Work out the finished part from the listing and answer in its coordinate system (mm). A direction names the side the tool comes from. Coordinates: 2 decimals unless noted, no trailing zeros. Write each loop counter-clockwise with the first axis right and the second up, starting at its lowest first coordinate (ties: lowest second). Pieces come first, ordered by that corner, then holes. Notation, with made-up numbers: (63, 78.25) - (79, 78.25) arc R11 cw to (79, 99.25) - close; hole circle Ø6 at (59.25, 89). An arc over 180 degrees is marked (long way). One line per item, written item: value.
Autodesk Inventor part; units mm, degrees
ref_plane "YZ Plane" through (0, 0, 0) normal (1, 0, 0) x (0, 1, 0)
ref_plane "XZ Plane" through (0, 0, 0) normal (0, 1, 0) x (-1, 0, 0)
ref_plane "XY Plane" through (0, 0, 0) normal (0, 0, 1) x (1, 0, 0)
sketch "Boceto1" plane through (0, 0, 0) normal (0, 0, 1) x (1, 0, 0)
  line L0 (0, 0) -> (0, 19.566)
  line L1 (2, 65) -> (2, 21)
  line L2 (2, 21) -> (0, 19.566)
  line L3 (2, 65) -> (14.5, 65)
  line L4 (29, 0) -> (29, 19.566)
  line L5 (27, 65) -> (27, 21)
  line L6 (27, 21) -> (29, 19.566)
  line L7 (27, 65) -> (14.5, 65)
  line L8 (0, 0) -> (29, 0)
extrude "Extrusión1" add sketch "Boceto1" along normal blind 7
sketch "Boceto2" plane through (0, 0, 7) normal (0, 0, 1) x (1, 0, 0)
  line L0 (27, 65) -> (27, 21)
  line L1 (2, 65) -> (27, 65)
  line L2 (2, 21) -> (2, 65)
  line L3 (2, 65) -> (5, 65)
  line L4 (2, 65) -> (2, 26)
  line L5 (5, 26) -> (5, 65)
  line L6 (27, 65) -> (24, 65)
  line L7 (24, 65) -> (24, 44)
  line L8 (27, 65) -> (27, 26)
  line L9 (5, 26) -> (2, 26)
  line L10 (24, 26) -> (27, 26)
  line L11 (24.1227, 26) -> (22, 26)
  line L12 (22, 26) -> (22, 44)
  line L13 (22, 44) -> (24, 44)
  dimension "d7" = 18
extrude "Extrusión2" add sketch "Boceto2" along normal blind 9
sketch "Boceto3" plane through (0, 0, 7) normal (0, 0, 1) x (1, 0, 0)
  line L0 (5, 65) -> (24, 65)
  line L1 (29, 0) -> (0, 0)
  line L2 (22, 44) -> (24, 44)
  line L3 (2, 0) -> (2, 21)
  line L4 (2, 21) -> (5, 21)
  line L5 (5, 21) -> (5, 0)
  line L6 (5, 0) -> (2, 0)
  line L7 (27, 0) -> (27, 21)
  line L8 (27, 21) -> (24, 21)
  line L9 (24, 21) -> (24, 0)
  line L10 (24, 0) -> (27, 0)
  dimension "d9" = 21
extrude "Extrusión3" add sketch "Boceto3" along normal blind 5
sketch "Boceto4" plane through (0, 0, 7) normal (0, 0, 1) x (1, 0, 0)
  line L0 (29, 0) -> (0, 0)
  line L1 (7, 10) -> (15, 10)
  line L2 (15, 10) -> (15, 27)
  line L3 (15, 27) -> (7, 27)
  line L4 (7, 27) -> (7, 10)
  dimension "d22" = 8
extrude "Extrusión4" add sketch "Boceto4" along normal blind 4
sketch "Sketch5" plane through (2, 65, 0) normal (0, 1, 0) x (1, 0, 0)
  line L0 (3, -7) -> (22, -7)
  line L1 (0, 0) -> (25, 0)
  line L2 (3, -7) -> (3, -16)
  line L3 (22, 2) -> (3, 2)
  line L4 (3, 2) -> (3, -2)
  line L5 (3, -2) -> (22, -2)
  line L6 (22, -2) -> (22, 2)
  line L7 (22, 2) -> (3, -2) construction
  line L8 (3, 2) -> (22, -2) construction
  line L9 (3, -2) -> (3, -7)
  line L10 (22, -7) -> (22, -2)
  line L11 (3, -7) -> (22, -7)
  point P0 (-2, 0)
  point P1 (12.5, 0)
  dimension "d23" = 4
extrude "Extrusion5" cut sketch "Sketch5" against normal up to surface (38 mm away) contours L9 L5 L10 L0
properties part number "fio"
Item 1: Determine the mould class of faces 5 (the face through (23, 44, 11)), 6 (the face through (14, 33, 0)), 7 (the face through (4, 26, 11)) for opening direction Y: +Y half, -Y half, draft (parallel to the pull), parting line (faces both ways), or undercut.
Evaluation:
face 5: +Y half
face 6: draft
face 7: undercut
Item 2: Which of the six approach directions +Z, -Z, +X, -X, +Y, -Y give full straight-line access (tool end or side, diameter ignored) to faces 1 (the face through (28, 11, 7)), 2 (the face through (2, 43, 8)), 3 (the face through (7, 19, 9)), 4 (the face through (3, 11, 12))?
Evaluation:
face 1: +Z, +X, +Y, -Y
face 2: +Z, -Z, -X, +Y
face 3: +Z, +Y, -Y
face 4: +Z, +X, -X, -Y
Item 3: Consider probe 1 along X at (y, z) = (13, 10.25); probe 2 along X at (y, z) = (58, 15); probe 3 along X at (y, z) = (37.5, 10). Determine where each line is inside the solid, lowest interval first.
Evaluation:
probe 1: x = 2 to 5, 7 to 15, 24 to 27
probe 2: x = 2 to 5, 24 to 27
probe 3: x = 2 to 5, 22 to 27
Item 4: Given pin 1 (3 mm diameter, centred on x = 17.5, z = 3, fed in from -Y); pin 2 (12 mm diameter, centred on x = 24, y = 13.5, fed in from +Z); pin 3 (2.5 mm diameter, centred on y = 15.5, z = 10.5, fed in from +X); pin 4 (4 mm diameter, centred on y = 11, z = 10.5, fed in from -X), each flat-ended and moving along its own axis, determine where each tip first touches the part or whether it passes through.
Evaluation:
pin 1: stops at y = 0
pin 2: stops at z = 12
pin 3: stops at x = 27
pin 4: stops at x = 2
Item 5: Section D-D, the plane y = 11.5 is taken. Determine the outline of the cut face in (x, z).
Evaluation:
outline: (0, 0) - (29, 0) - (29, 7) - (27, 7) - (27, 12) - (24, 12) - (24, 7) - (15, 7) - (15, 11) - (7, 11) - (7, 7) - (5, 7) - (5, 12) - (2, 12) - (2, 7) - (0, 7) - close
Item 6: Section B-B, the plane z = 13.25 is taken. Determine the outline of the cut face in (x, y).
Evaluation:
outline: (2, 26) - (5, 26) - (5, 65) - (2, 65) - close; (22, 26) - (27, 26) - (27, 65) - (24, 65) - (24, 44) - (22, 44) - close
Item 7: Section A-A, the plane z = 8.5 is taken. Determine the outline of the cut face in (x, y), then the cut area to 3 significant figures.
Evaluation:
outline: (2, 0) - (5, 0) - (5, 21) - (2, 21) - close; (2, 26) - (5, 26) - (5, 65) - (2, 65) - close; (7, 10) - (15, 10) - (15, 27) - (7, 27) - close; (22, 26) - (27, 26) - (27, 65) - (24, 65) - (24, 44) - (22, 44) - close; (24, 0) - (27, 0) - (27, 21) - (24, 21) - close
area: 532 mm2
Item 8: Section C-C, the plane x = 11 is taken. Determine the outline of the cut face in (y, z), then the cut area to 3 significant figures.
Evaluation:
outline: (0, 0) - (65, 0) - (65, 2) - (27, 2) - (27, 11) - (10, 11) - (10, 7) - (0, 7) - close
area: 333 mm2
